The drawing under review shows one solid part. Ordinate dimensions are in mm from its lowest x, y, z. A direction names the side the tool comes from. Give positions to 0.01 mm unless a question says otherwise; leave off trailing zeros. Loops run counter-clockwise (first coordinate to the right, second up) from the corner with the lowest first, then second, coordinate; pieces in that order, holes last. Notation, with made-up numbers: (0, -11.75) -> (59, -11.75) arc R6 cw to (59, -5.75) -> close; hole circle Ø7 at (8, 45). An arc over 180 degrees is marked (long way). Answer in a Markdown table with one row per item. Add a question column.
(1) For the marked faces 3 and 4, list the 3-axis set-ups (+Z, -Z, +X, -X, +Y, -Y) from which the entire face can be reached by the end or side of a thin tool; tool diameter is ignored.
(2) Draft analysis for pull direction Z (two halves, no side actions). For the marked faces 1 and 2, state which applies: +Z half, -Z half, draft (parallel to the pull), parting line (faces both ways), or undercut.
(3) Consider section A-A on y = 31. Write out the cut boundary in (x, z), then the cut area to 3 significant figures.
(4) Consider section B-B on z = 16.5. Write out the cut boundary in (x, y).
(5) For line 1 (Z direction, x = 71.5, y = 7.5); line 2 (X direction, y = 22, z = 48); line 3 (Y direction, x = 102.5, z = 36), list the stretches that pass through material, from the lowest coordinate up.
(6) Consider section D-D on z = 47. Write out the cut boundary in (x, y), then the cut area to 3 significant figures.
(7) Consider section C-C on x = 124. Write out the cut boundary in (y, z), then the cut area to 3 significant figures.
(8) For pin 1 (2.5 mm diameter, centred on x = 145.5, y = 24, fed in from -Z); pin 2 (4 mm diameter, centred on x = 102.5, y = 11.5, fed in from +Z); pin 3 (24 mm diameter, centred on x = 68, z = 43.5, fed in from +Y); pin 4 (2.5 mm diameter, centred on x = 146, y = 19.5, fed in from +Z), all flat-tipped, find the tip position at first contact; note any pin that passes through.
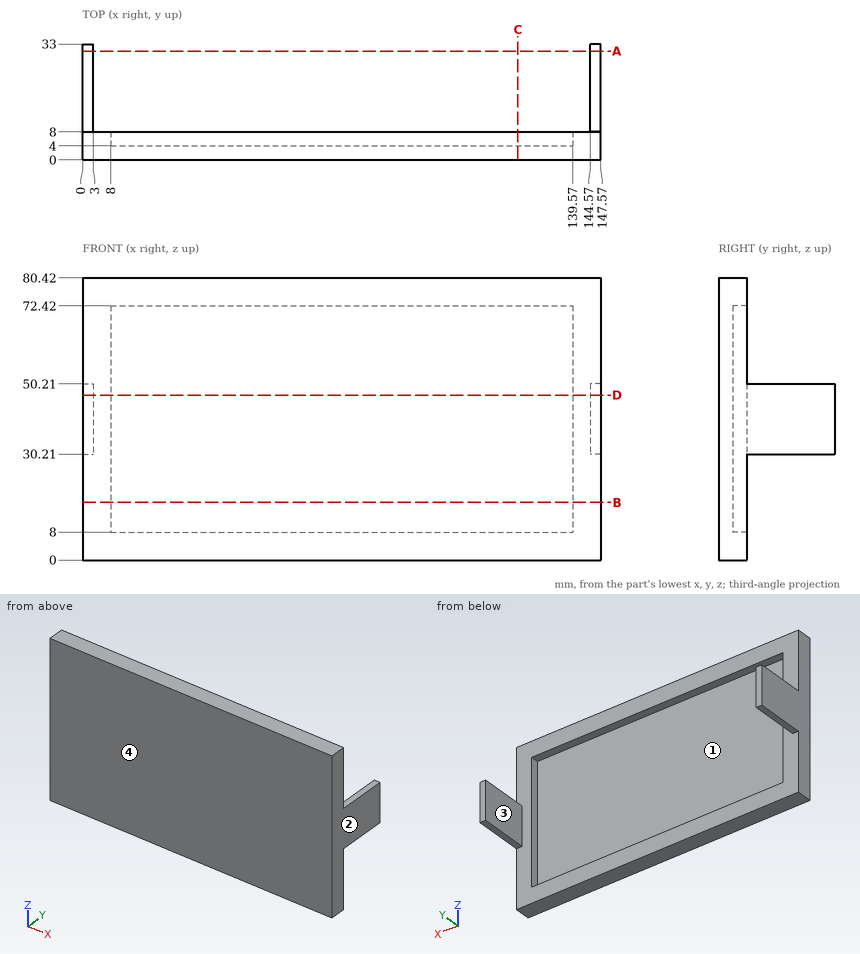
Values follow:
| question | item | result |
|---|---|---|
| 1 | face 3 | +Z, -Z, +Y |
| 1 | face 4 | +Z, -Z, +X, -X, -Y |
| 2 | face 1 | undercut |
| 2 | face 2 | draft |
| 3 | outline | (0, 30.21) -> (3, 30.21) -> (3, 50.21) -> (0, 50.21) -> close; (144.57, 30.21) -> (147.57, 30.21) -> (147.57, 50.21) -> (144.57, 50.21) -> close |
| 3 | area | 120 mm2 |
| 4 | outline | (0, 0) -> (147.57, 0) -> (147.57, 8) -> (139.57, 8) -> (139.57, 4) -> (8, 4) -> (8, 8) -> (0, 8) -> close |
| 5 | line 1 | 0 to 8, 72.42 to 80.42 |
| 5 | line 2 | 0 to 3, 144.57 to 147.57 |
| 5 | line 3 | 0 to 4 |
| 6 | outline | (0, 0) -> (147.57, 0) -> (147.57, 33) -> (144.57, 33) -> (144.57, 8) -> (139.57, 8) -> (139.57, 4) -> (8, 4) -> (8, 8) -> (3, 8) -> (3, 33) -> (0, 33) -> close |
| 6 | area | 804 mm2 |
| 7 | outline | (0, 0) -> (8, 0) -> (8, 8) -> (4, 8) -> (4, 72.42) -> (8, 72.42) -> (8, 80.42) -> (0, 80.42) -> close |
| 7 | area | 386 mm2 |
| 8 | pin 1 | z = 30.21 |
| 8 | pin 2 | through |
| 8 | pin 3 | y = 4 |
| 8 | pin 4 | z = 50.21 |
